Geometry check sheet. Reference: the model listing, model coordinates, mm. A direction names the side the tool comes from. Coordinates: 2 decimals unless noted, no trailing zeros. Loops run counter-clockwise (first coordinate to the right, second up) from the corner with the lowest first, then second, coordinate; pieces in that order, holes last.
Autodesk Inventor part; units mm, degrees
ref_plane "YZ Plane" through (0, 0, 0) normal (1, 0, 0) x (0, 1, 0)
ref_plane "XZ Plane" through (0, 0, 0) normal (0, 1, 0) x (-1, 0, 0)
ref_plane "XY Plane" through (0, 0, 0) normal (0, 0, 1) x (1, 0, 0)
sketch "Sketch1" plane through (0, 0, 0) normal (0, 0, 1) x (1, 0, 0)
  line L0 (0, 0) -> (38.1, 0)
  line L1 (38.1, 0) -> (38.1, -50.8)
  line L2 (38.1, -50.8) -> (34.925, -50.8)
  line L3 (34.925, -50.8) -> (34.925, -3.175)
  line L4 (34.925, -3.175) -> (0, -3.175)
  line L5 (0, -3.175) -> (0, 0)
  dimension "d0" = 50.8
  dimension "d1" = 38.1
  dimension "d2" = 3.175
  dimension "d3" = 3.175
extrude "Extrusion1" add sketch "Sketch1" along normal blind 203.2
sketch "Sketch2" plane through (0, -3.175, 0) normal (0, 1, 0) x (1, 0, 0)
  line L0 (38.1, -203.2) -> (0, -203.2)
  line L1 (38.1, 0) -> (38.1, -203.2)
  line L2 (0, 0) -> (0, -203.2)
  line L3 (0, 0) -> (38.1, 0)
  point P0 (25.2222, -153.4922)
  point P1 (9.9314, -139.0904)
  point P2 (25.2222, -80.4672)
  point P3 (9.9314, -66.0654)
  point P4 (25.2222, -42.3672)
  point P5 (9.9314, -27.9654)
  dimension "d6" = 49.7078
  dimension "d8" = 9.9314
  dimension "d9" = 64.1096
  dimension "d10" = 25.2222
  dimension "d11" = 80.4672
  dimension "d12" = 25.2222
  dimension "d13" = 66.0654
  dimension "d14" = 9.9314
  dimension "d15" = 42.3672
  dimension "d16" = 25.2222
  dimension "d17" = 27.9654
  dimension "d18" = 9.9314
hole "Hole1" at (25.2222, -3.175, 153.4922) at (9.9314, -3.175, 139.0904) at (25.2222, -3.175, 80.4672) at (9.9314, -3.175, 66.0654) at (25.2222, -3.175, 42.3672) at (9.9314, -3.175, 27.9654) direction (0, 1, 0) diameter 5.1054 end through all countersink diameter 9.525 countersink angle 82
sketch "Sketch4" plane through (34.925, -50.8, 0) normal (1, 0, 0) x (0, 0, -1)
  line L0 (0, 50.8) -> (0, 0)
  line L1 (0, 50.8) -> (-203.2, 50.8)
  line L2 (-203.2, 0) -> (-203.2, 50.8)
  point P0 (-22.225, 34.925)
  point P1 (-22.225, 9.525)
  point P2 (-155.575, 34.925)
  point P3 (-155.575, 9.525)
  point P4 (-111.125, 34.925)
  point P5 (-111.125, 9.525)
  dimension "d29" = 25.4
  dimension "d30" = 22.225
  dimension "d31" = 22.225
  dimension "d32" = 15.875
  dimension "d33" = 47.625
  dimension "d34" = 47.625
  dimension "d35" = 25.4
  dimension "d36" = 15.875
  dimension "d41" = 92.075
  dimension "d42" = 92.075
  dimension "d43" = 25.4
  dimension "d44" = 15.875
hole "Hole2" at (34.925, -15.875, 22.225) at (34.925, -41.275, 22.225) at (34.925, -15.875, 155.575) at (34.925, -41.275, 155.575) at (34.925, -15.875, 111.125) at (34.925, -41.275, 111.125) direction (1, 0, 0) diameter 5.1054 end through all countersink diameter 9.779 countersink angle 82
sketch "Sketch5" plane through (34.925, -50.8, 0) normal (-1, 0, 0) x (0, 0, 1)
  line L0 (0, 47.625) -> (203.2, 47.625)
  line L1 (0, 0) -> (0, 47.625)
  point P0 (0, 50.8)
  point P1 (38.1, 34.925)
  point P2 (95.25, 34.925)
  point P3 (185.7899, 34.925)
  dimension "d52" = 12.7
  dimension "d53" = 38.1
  dimension "d54" = 95.25
  dimension "d55" = 185.7899
hole "Hole3" at (34.925, -15.875, 38.1) at (34.925, -15.875, 95.25) at (34.925, -15.875, 185.7899) direction (1, 0, 0) diameter 6.35 end through all
equation "\"d3\" = d2"
properties part number "CLB_086_ClimberMountLowerAngle" material "Aluminum 6061"
(1) Sectioned sample at B-B on z = 178.5. Record the cut outline in (x, y) (3 decimals).
Findings:
outline: (0, -3.175) - (34.925, -3.175) - (34.925, -50.8) - (38.1, -50.8) - (38.1, 0) - (0, 0) - close
(2) Sectioned sample at C-C on y = -7. Record the cut outline in (x, z) (3 decimals).
Findings:
outline: (34.925, 0) - (38.1, 0) - (38.1, 203.2) - (34.925, 203.2) - close
(3) Scan lines: L1, parallel to X at y = -11, z = 62.5 (3 decimals); L2, parallel to Y at x = 22.5, z = 133.5 (3 decimals); L3, parallel to X at y = -12, z = 21.5. Record each from-to range of solid material in increasing order.
Findings:
L1: x = 34.925 to 38.1
L2: y = -3.175 to 0
L3: x = 36.01 to 38.1
(4) Access from +Z, -Z, +X, -X, +Y, -Y to the whole of each face (thin tool, end or side, straight path). Record for faces 5 (the flat face through (34.925, -27, 100)), 6 (the conical face through (26.03, -0.79, 77.9)).
Findings:
face 5: +Z, -Z, -X, -Y
face 6: -Y
(5) Gauge pin test, flat ends, axial feed: pin 1 Ø7.5 at (y, z) = (-15.875, 95.25) entering from +X; pin 2 Ø6.5 at (x, z) = (25.22, 153.49) entering from -Y; pin 3 Ø10.5 at (x, z) = (10, 146.5) entering from -Y (3 decimals); pin 4 Ø10 at (y, z) = (-32.5, 77.5) entering from -X (3 decimals). Record the tip position at first contact, or that the pin passes through.
Findings:
pin 1: stops at x = 38.1
pin 2: stops at y = -1.44
pin 3: stops at y = -3.175
pin 4: stops at x = 34.925
(6) Draft check along Z on faces 1 (the conical face through (37.445, -15.756, 108.429)), 2 (the conical face through (37.45, -39.45, 20.24)), 3 (the flat face through (36, -14, 203.2)), 4 (the flat face through (18, -3.175, 100)). Enter one of: +Z half, -Z half, draft (parallel to the pull), parting line (faces both ways), or undercut.
Findings:
face 1: undercut
face 2: undercut
face 3: +Z half
face 4: draft
(7) Sectioned sample at A-A on z = 95.25. Record the cut outline in (x, y) (3 decimals), and give its area (3 significant figures).
Findings:
outline: (0, -3.175) - (34.925, -3.175) - (34.925, -12.7) - (38.1, -12.7) - (38.1, 0) - (0, 0) - close; (34.925, -50.8) - (38.1, -50.8) - (38.1, -19.05) - (34.925, -19.05) - close
area: 252 mm2
